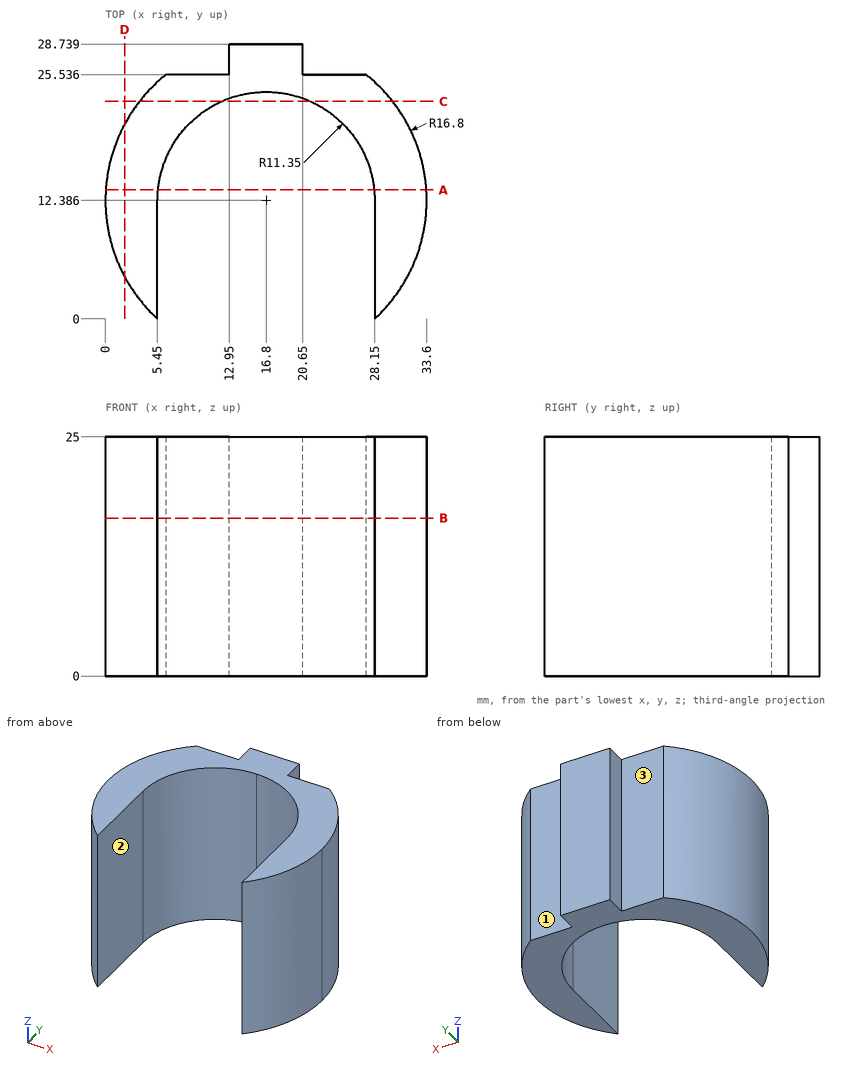
Drawing for the job (mm, zero at the part's lowest x, y, z). A direction names the side the tool comes from. Give positions to 0.01 mm unless a question says otherwise; leave off trailing zeros. Order: outer loops, then holes, each group sorted by start corner. A loop starts at its lowest first (then second) coordinate and runs counter-clockwise, first axis right, second up. Notation, with made-up numbers: M -22,55 L 1,55 A24 cw 1,71 Z; hole C -27.5,-20.75 d1. An arc over 180 degrees is marked long. Use a Markdown table: item, result. Add a question column.
(1) Saw through at C-C, the plane y = 22.75. Give the cut face in (x, z), and give its area (3 significant figures).
(2) Saw through at B-B, the plane z = 16.5. Give the cut face in (x, y), and give its area (3 significant figures).
(3) Saw through at A-A, the plane y = 13.5. Give the cut face in (x, z) (1 decimal).
(4) Drop flat-ended pins along their axis: P1, Ø1, axis at y = 27, z = 12.5, coming from the +X side; P2, Ø3, axis at x = 7, y = 12, coming from the -Z side; P3, Ø3.5, axis at y = 6, z = 18, coming from the +X side; P4, Ø3.5, axis at y = 8, z = 16.5, coming from the -X side. Give the stop position or say it passes through.
(5) Saw through at D-D, the plane x = 2. Give the cut face in (y, z), and give its area (4 significant figures).
(6) Probe line 1 along Y through (x, z) = (17, 12.5); line 2 along X through (y, z) = (10.5, 1.25); line 3 along X through (y, z) = (12.5, 17). List the from-to ranges inside material, lowest first. Write a range as [from, to].
(7) 3-axis set-ups, long thin cutter, end or side, ignore diameter. For the marked faces 1, 2 and 3: which of +Z, -Z, +X, -X, +Y, -Y reach the whole face in a straight line?
Answer key:
| question | item | result |
|---|---|---|
| 1 | outline | M 3.58,0 L 12.17,0 L 12.17,25 L 3.58,25 Z; M 21.43,0 L 30.02,0 L 30.02,25 L 21.43,25 Z |
| 1 | area | 430 mm^2 |
| 2 | outline | M 5.45,0 L 5.45,12.39 A11.35 cw 28.15,12.39 L 28.15,0 A16.8 ccw 33.6,12.39 A16.8 ccw 27.26,25.54 L 20.65,25.54 L 20.65,28.74 L 12.95,28.74 L 12.95,25.54 L 6.34,25.54 A16.8 ccw Z |
| 2 | area | 307 mm^2 |
| 3 | outline | M 0,0 L 5.5,0 L 5.5,25 L 0,25 Z; M 28.1,0 L 33.6,0 L 33.6,25 L 28.1,25 Z |
| 4 | P1 | x = 20.65 |
| 4 | P2 | through |
| 4 | P3 | x = 32.95 |
| 4 | P4 | x = 0.21 |
| 5 | outline | M 4.44,0 L 20.34,0 L 20.34,25 L 4.44,25 Z |
| 5 | area | 397.5 mm^2 |
| 6 | line 1 | [23.73, 28.74] |
| 6 | line 2 | [0.11, 5.45], [28.15, 33.49] |
| 6 | line 3 | [0, 5.45], [28.15, 33.6] |
| 7 | face 1 | +Z, -Z, +X, +Y |
| 7 | face 2 | +Z, -Z, -Y |
| 7 | face 3 | +Z, -Z, -X, +Y |
